Check sheet for the modelled part. Datum: model origin and axes. Units: mm. A direction names the side the tool comes from. Give positions to 0.01 mm unless a question says otherwise; leave off trailing zeros. Write each loop counter-clockwise with the first axis right and the second up, starting at its lowest first coordinate (ties: lowest second). Pieces come first, ordered by that corner, then holes. Notation, with made-up numbers: M -24,-36.5 L 29,-36.5 A7 cw 29,-31.5 Z; hole C 13,34 d8. An arc over 180 degrees is marked long. Write item = value, one per line. Start each with the question number.
1) Draft check along Y on faces 1 (the face through (4, 95, 101)), 2 (the face through (-1, -100, 99)), 3 (the face through (-97, 0, 200)). Enter one of: pulls with the +Y half, pulls with the -Y half, needs draft (parallel to the pull), parting line crosses it, or undercut.
2) Set-up check for faces 4 (the face through (-95, 1, 101)), 5 (the face through (100, 0, -2)): record each of +Z, -Z, +X, -X, +Y, -Y from which the full face is reachable in a straight line by a thin tool's end or side.
3) Sectioned sample at C-C, the plane y = 83.5. Record the cut outline in (x, z), then the cut area to 3 significant figures.
4) Scan lines: L1, parallel to Y at x = -87, z = 140; L2, parallel to X at y = 32, z = 73; L3, parallel to Z at x = 74, y = -7.5. Record each from-to range of solid material in increasing order.
5) Gauge pin test, flat ends, axial feed: pin 1 (3 mm diameter, centred on y = 47.5, z = 33.5, fed in from +X); pin 2 (6 mm diameter, centred on x = 13, y = 52, fed in from +Z). Record the tip position at first contact, or that the pin passes through.
6) Sectioned sample at A-A, the plane x = -47.5. Record the cut outline in (y, z), then the cut area to 3 significant figures.
7) Sectioned sample at B-B, the plane z = 69. Record the cut outline in (x, y).
from build123d import *

# Parameters (mm, degrees)
F0_W     = 200
F0_H     = 200
F5_DEPTH = 5
F1_W     = 200
F1_H     = 200
F6_DEPTH = 5
F2_W     = 200
F2_H     = 200
F3_DEPTH = 5
F4_W     = 190
F4_H     = 200
F7_DEPTH = 5


with BuildPart() as f5:
    # F0 (on Top) → F5 (new body)
    with BuildSketch(Plane.XY):
        Rectangle(F0_W, F0_H)
    extrude(amount=-F5_DEPTH)

    # F1 (on face) → F6 (join)
    with BuildSketch(Plane.XZ.offset(100)):
        with Locations((0, 100)):
            Rectangle(F1_W, F1_H)
    extrude(amount=-F6_DEPTH)

    # F2 (on face) → F3 (join)
    with BuildSketch(Plane(origin=(0, 100, 0), x_dir=(-1, 0, 0), z_dir=(0, 1, 0))):
        with Locations((0, 100)):
            Rectangle(F2_W, F2_H)
    extrude(amount=-F3_DEPTH)

    # F4 (on face) → F7 (join)
    with BuildSketch(Plane(origin=(-100, 0, 0), x_dir=(0, -1, 0), z_dir=(-1, 0, 0))):
        with Locations((0, 100)):
            Rectangle(F4_W, F4_H)
    extrude(amount=-F7_DEPTH)


solid = f5.part
Data:
q1.face_1 = undercut
q1.face_2 = pulls with the -Y half
q1.face_3 = needs draft
q2.face_4 = +Z, +X
q2.face_5 = +Z, -Z, +X, +Y, -Y
q3.outline = M -100,-5 L 100,-5 L 100,0 L -95,0 L -95,200 L -100,200 Z
q3.area = 2,000 mm2
q4.L1 = -100 to -95, 95 to 100
q4.L2 = -100 to -95
q4.L3 = -5 to 0
q5.pin_1 = -95
q5.pin_2 = 0
q6.outline = M -100,-5 L 100,-5 L 100,200 L 95,200 L 95,0 L -95,0 L -95,200 L -100,200 Z
q6.area = 3,000 mm2
q7.outline = M -100,-100 L 100,-100 L 100,-95 L -95,-95 L -95,95 L 100,95 L 100,100 L -100,100 Z
